Read the model definition and answer for the solid it produces. Units are mm, in the model's axes. Face numbers are marked on the shaded views. A direction names the side the tool comes from. Coordinates: 2 decimals unless noted, no trailing zeros. Write each loop counter-clockwise with the first axis right and the second up, starting at its lowest first coordinate (ties: lowest second). Pieces come first, ordered by that corner, then holes. Notation, with made-up numbers: (50, 25.25) -> (74, 25.25) arc R8 cw to (74, 31.25) -> close; hole circle Ø7 at (53, 85.25). An arc over 180 degrees is marked (long way). Use CSV: the item, a comma, the result in double quotes. Start each with the question number.
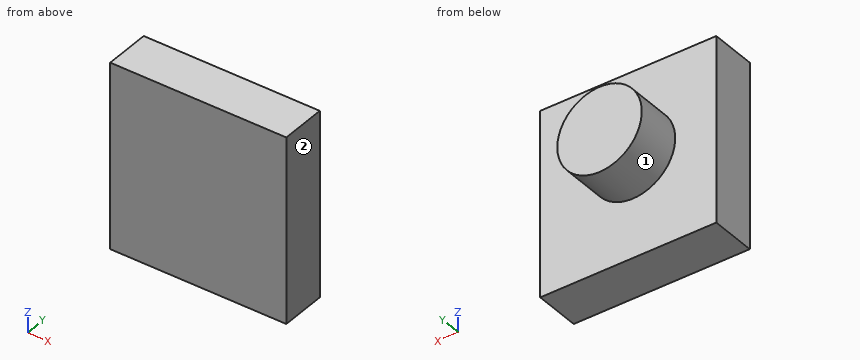
Autodesk Inventor part; units mm, degrees
ref_plane "YZ Plane" through (0, 0, 0) normal (1, 0, 0) x (0, 1, 0)
ref_plane "XZ Plane" through (0, 0, 0) normal (0, 1, 0) x (-1, 0, 0)
ref_plane "XY Plane" through (0, 0, 0) normal (0, 0, 1) x (1, 0, 0)
sketch "Sketch1" plane through (0, 0, 0) normal (0, 1, 0) x (-1, 0, 0)
  line L0 (0, 0) -> (9.7707, 0)
  line L1 (9.7707, 0) -> (9.7707, -10.2745)
  line L2 (9.7707, -10.2745) -> (0, -10.2745)
  line L3 (0, -10.2745) -> (0, 0)
extrude "Extrusion1" add sketch "Sketch1" along normal blind 2.54
sketch "Sketch2" plane through (0, 2.54, 0) normal (0, 1, 0) x (1, 0, 0)
  circle A0 centre (-5.1463, 4.6604) radius 2.3446
  point P0 (0, 0)
extrude "Extrusion2" add sketch "Sketch2" along normal blind 2.54
properties part number "offset_sketch_plane"
1) Section A-A, the plane x = -5 is taken. Give the vertices of the cut face in (y, z), plus the area to 3 significant figures.
2) Find the intervals of material crossed by line 1 along Y through (x, z) = (-7.25, -2.5); line 2 along X through (y, z) = (4.35, -4.75); line 3 along Z through (x, y) = (-3.5, 2.7), in increasing order.
3) Section C-C, the plane y = 3.9 is taken. Give the vertices of the cut face in (x, z), plus the area to 3 significant figures.
4) Which of the six approach directions +Z, -Z, +X, -X, +Y, -Y give full straight-line access (tool end or side, diameter ignored) to the marked faces 1 and 2?
5) Section D-D, the plane x = -8 is taken. Give the vertices of the cut face in (y, z).
6) Section B-B, the plane z = -4.5 is taken. Give the vertices of the cut face in (x, y).
The answers:
1,outline,"(0, -10.27) -> (2.54, -10.27) -> (2.54, -7) -> (5.08, -7) -> (5.08, -2.32) -> (2.54, -2.32) -> (2.54, 0) -> (0, 0) -> close"
1,area,"38.0 mm^2"
2,line 1,"y = 0 to 2.54"
2,line 2,"x = -7.49 to -2.8"
2,line 3,"z = -6.33 to -2.99"
3,outline,"circle Ø4.69 at (-5.15, -4.66)"
3,area,"17.3 mm^2"
4,face 1,"+Y"
4,face 2,"+Z, -Z, +X, +Y, -Y"
5,outline,"(0, -10.27) -> (2.54, -10.27) -> (2.54, 0) -> (0, 0) -> close"
6,outline,"(-9.77, 0) -> (0, 0) -> (0, 2.54) -> (-2.81, 2.54) -> (-2.81, 5.08) -> (-7.49, 5.08) -> (-7.49, 2.54) -> (-9.77, 2.54) -> close"
